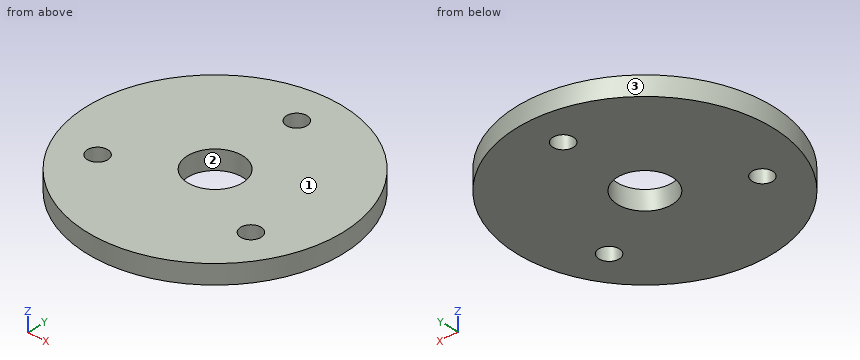
Autodesk Inventor part; units mm, degrees
ref_plane "YZ Plane" through (0, 0, 0) normal (1, 0, 0) x (0, 1, 0)
ref_plane "XZ Plane" through (0, 0, 0) normal (0, 1, 0) x (-1, 0, 0)
ref_plane "XY Plane" through (0, 0, 0) normal (0, 0, 1) x (1, 0, 0)
sketch "Sketch1" plane through (0, 0, 0) normal (0, 0, 1) x (1, 0, 0)
  circle A0 centre (0, 0) radius 20
  circle A1 centre (0, 0) radius 4.3
  dimension "d0" = 40
  dimension "d2" = 8.6
extrude "Extrusion1" add sketch "Sketch1" along normal blind 3
sketch "Sketch2" plane through (0, 0, 3) normal (0, 0, 1) x (1, 0, 0)
  circle A0 centre (0, 14) radius 1.6
  line L0 (0, -28) -> (0, 28)
  point P0 (0, 0)
  dimension "d5" = 14
  dimension "d6" = 3.2
extrude "Extrusion2" cut sketch "Sketch2" against normal blind 10
pattern_circular "Circular Pattern1" count 3 over 360 about axis through (0, 0, 0) along (0, 0, 1) of "Extrusion2"
properties part number "bearing_holder"
The model under review builds one solid part; all positions refer to its coordinate system, in mm. Face numbers are marked on the shaded views. Round coordinates to 2 decimals unless told otherwise and drop trailing zeros. Loops run counter-clockwise (first coordinate to the right, second up) from the corner with the lowest first, then second, coordinate; pieces in that order, holes last. Notation, with made-up numbers: (-36, 53) -> (-2, 53) arc R18 ccw to (-2, 63) -> close; hole circle Ø9 at (67.25, -27.75). An arc over 180 degrees is marked (long way). Answer as a JSON object with one key per item and string values. Group by question number.
1) For pin 1 Ø14 at (x, y) = (0, 0) entering from -Z; pin 2 Ø1 at (x, z) = (-8, 1) entering from -Y, all flat-tipped, find the tip position at first contact; note any pin that passes through.
2) We need section B-B on x = 0. Write out the cut boundary in (y, z).
3) For line 1 (Y direction, x = 0, z = 1.75); line 2 (Y direction, x = -0.5, z = 2.55); line 3 (X direction, y = 3, z = 1.65), list the stretches that pass through material, from the lowest coordinate up. Write a range as [from, to].
4) Mouldability with a two-part tool opening along Y and no side actions: class the marked faces 1, 2 and 3 as released by +Y, released by -Y, zero draft, split by the parting line, or undercut.
5) We need section C-C on y = -7. Write out the cut boundary in (x, z) (3 decimals), then the cut area to 3 significant figures.
6) We need section D-D on x = 13. Write out the cut boundary in (y, z), then the cut area to 3 significant figures.
7) We need section A-A on y = 0. Write out the cut boundary in (x, z), then the cut area to 3 significant figures.
Result set:
{
 "1": {"pin 1": "z = 0", "pin 2": "y = -18.54"},
 "2": {"outline": "(-20, 0) -> (-4.3, 0) -> (-4.3, 3) -> (-20, 3) -> close; (4.3, 0) -> (12.4, 0) -> (12.4, 3) -> (4.3, 3) -> close; (15.6, 0) -> (20, 0) -> (20, 3) -> (15.6, 3) -> close"},
 "3": {"line 1": "[-20, -4.3], [4.3, 12.4], [15.6, 20]", "line 2": "[-19.99, -4.27], [4.27, 12.48], [15.52, 19.99]", "line 3": "[-19.77, -3.08], [3.08, 19.77]"},
 "4": {"face 1": "zero draft", "face 2": "undercut", "face 3": "split by the parting line"},
 "5": {"outline": "(-18.735, 0) -> (-13.724, 0) -> (-13.724, 3) -> (-18.735, 3) -> close; (-10.524, 0) -> (10.524, 0) -> (10.524, 3) -> (-10.524, 3) -> close; (13.724, 0) -> (18.735, 0) -> (18.735, 3) -> (13.724, 3) -> close", "area": "93.2 mm²"},
 "6": {"outline": "(-15.2, 0) -> (-8.34, 0) -> (-8.34, 3) -> (-15.2, 3) -> close; (-5.66, 0) -> (15.2, 0) -> (15.2, 3) -> (-5.66, 3) -> close", "area": "83.2 mm²"},
 "7": {"outline": "(-20, 0) -> (-4.3, 0) -> (-4.3, 3) -> (-20, 3) -> close; (4.3, 0) -> (20, 0) -> (20, 3) -> (4.3, 3) -> close", "area": "94.2 mm²"}
}
